The model under review builds one solid part; all positions refer to its coordinate system, in mm. A direction names the side the tool comes from. Round coordinates to 2 decimals unless told otherwise and drop trailing zeros. Write each loop counter-clockwise with the first axis right and the second up, starting at its lowest first coordinate (ties: lowest second). Pieces come first, ordered by that corner, then holes. Notation, with made-up numbers: (70, 32) -> (122, 32) arc R16 ccw to (122, 49) -> close; hole circle Ø1 at (-33, -4.75). An arc over 180 degrees is marked (long way). Use CSV: the item, a comma, the result in double quotes. Start each with the question number.
1) Take a section at C-C, the plane y = 2.5. Give the boundary of the cut face in (x, z), then the cut area to 3 significant figures.
2) Take a section at A-A, the plane x = 0. Give the boundary of the cut face in (y, z), then the cut area to 3 significant figures.
3) For pin 1 Ø1 at (y, z) = (3, 1) entering from +X; pin 2 Ø1.5 at (x, y) = (-2, 2.5) entering from -Z, all flat-tipped, find the tip position at first contact; note any pin that passes through.
4) Wall thickness on probe 1 along Z at (x, y) = (-0.1, 3); probe 2 along Y at (x, z) = (-2.05, -0.3); probe 3 along Z at (x, y) = (1.35, 4.5): over which ranges is each line inside the solid? List them lowest first. Write a range as [from, to].
5) Take a section at B-B, the plane z = 0. Give the boundary of the cut face in (x, y), then the cut area to 3 significant figures.
6) Machinability: for faces 1 (the face through (2, -5.5, 1)), 2 (the face through (0, -7.5, 0)), which of the approach directions +Z, -Z, +X, -X, +Y, -Y give a long, thin tool a straight path to every point of the face, cutting with its end or side? Answer none if there is none.
from build123d import *

# Parameters (mm, degrees)
SKETCH_1_R      = 2
EXTRUDE_1_DEPTH = 6.5
EXTRUDE_START   = 1
SKETCH_2_R      = 2.5
EXTRUDE_2_DEPTH = 2


# Read off the part's stored shape, not the designer's step: M4 机械螺纹 螺柱1
with BuildPart() as part:
    # 草图1 → 凸台-拉伸1 (new, symmetric)
    with BuildSketch(Plane(origin=(0, 0, 0), x_dir=(1, 0, 0), z_dir=(0, 1, 0))):
        with Locations(Location((0, 0, 0), (0, 0, 90))):
            Circle(SKETCH_1_R)
    extrude(amount=EXTRUDE_1_DEPTH, both=True)

    # 草图2 → 凸台-拉伸2 (add)
    with BuildSketch(Plane.XZ.offset(6.5).offset(EXTRUDE_START)):
        with Locations(Location((0, 0, 0), (0, 0, 270))):
            Circle(SKETCH_2_R)
    extrude(amount=-EXTRUDE_2_DEPTH)

    # M4 机械螺纹 螺柱1 outline → M4 机械螺纹 螺柱1 (revolve, cut)
    with BuildSketch(Plane.XY):
        Polygon((2, 6.5), (1.621, 6.5), (2, 6.121), align=None)
    revolve(axis=Axis((0, 0, 0), (0, 1, 0)), mode=Mode.SUBTRACT)


solid = part.part
Values found:
1,outline,"circle Ø4 at (0, 0)"
1,area,"12.6 mm²"
2,outline,"(-7.5, -2.5) -> (-5.5, -2.5) -> (-5.5, -2) -> (6.12, -2) -> (6.5, -1.62) -> (6.5, 1.62) -> (6.12, 2) -> (-5.5, 2) -> (-5.5, 2.5) -> (-7.5, 2.5) -> close"
2,area,"57.9 mm²"
3,pin 1,"x = 1.94"
3,pin 2,"z = -1.56"
4,probe 1,"[-2, 2]"
4,probe 2,"[-7.5, -5.5]"
4,probe 3,"[-1.48, 1.48]"
5,outline,"(-2.5, -7.5) -> (2.5, -7.5) -> (2.5, -5.5) -> (2, -5.5) -> (2, 6.12) -> (1.62, 6.5) -> (-1.62, 6.5) -> (-2, 6.12) -> (-2, -5.5) -> (-2.5, -5.5) -> close"
5,area,"57.9 mm²"
6,face 1,"+Y"
6,face 2,"+Z, -Z, +X, -X, -Y"
